The model under review builds one solid part; all positions refer to its coordinate system, in mm. A direction names the side the tool comes from. Coordinates: 2 decimals unless noted, no trailing zeros. Write each loop counter-clockwise with the first axis right and the second up, starting at its lowest first coordinate (ties: lowest second). Pieces come first, ordered by that corner, then holes. Notation, with made-up numbers: M -37,10.25 L 22,10.25 A15 ccw 22,18.25 Z; hole C 24,28 d9. An arc over 180 degrees is marked long. Answer as CSV lines item,"result". Start each with the question number.
Autodesk Inventor part; units mm, degrees
ref_plane "YZ Plane" through (0, 0, 0) normal (1, 0, 0) x (0, 1, 0)
ref_plane "XZ Plane" through (0, 0, 0) normal (0, 1, 0) x (-1, 0, 0)
ref_plane "XY Plane" through (0, 0, 0) normal (0, 0, 1) x (1, 0, 0)
sketch "Szkic1" plane through (0, 0, 0) normal (0, 1, 0) x (-1, 0, 0)
  line L0 (1.5, 2) -> (-1.5, 2)
  line L1 (-1.5, 2) -> (-1.5, -2)
  line L2 (-1.5, -2) -> (1.5, -2)
  line L3 (1.5, -2) -> (1.5, 2)
  line L4 (1.5, 2) -> (-1.5, -2) construction
  line L5 (-1.5, 2) -> (1.5, -2) construction
  point P0 (0, 0)
  dimension "d0" = 4
  dimension "d1" = 3
extrude "Wyciągnięcie proste1" add sketch "Szkic1" along normal blind 26.5
sketch "Szkic2" plane through (-1.5, 0, -2) normal (-1, 0, 0) x (0, 0, 1)
  line L0 (4, 26.5) -> (0, 26.5)
  line L1 (4, 0) -> (4, 26.5)
  line L2 (0, 26.5) -> (4, 26.5)
  line L3 (4, 26.5) -> (4, 22.5)
  line L4 (4, 22.5) -> (0, 22.5)
  line L5 (0, 22.5) -> (0, 26.5)
  point P0 (2, 0)
  dimension "d4" = 4
extrude "Wyciągnięcie proste2" add sketch "Szkic2" along normal blind 15.5
sketch "Szkic3" plane through (-1.5, 22.5, -2) normal (0, -1, 0) x (1, 0, 0)
  line L0 (3, 4) -> (-15.5, 4)
  line L1 (3, 0) -> (-15.5, 0)
  line L2 (-15.5, 4) -> (-12.5, 4)
  line L3 (-12.5, 4) -> (-12.5, 0)
  line L4 (-12.5, 0) -> (-15.5, 0)
  line L5 (-15.5, 0) -> (-15.5, 4)
  point P0 (1.5, 2)
  dimension "d7" = 3
extrude "Wyciągnięcie proste3" add sketch "Szkic3" along normal blind 22.5
sketch "Szkic4" plane through (1.5, 0, 2) normal (1, 0, 0) x (0, 0, -1)
  line L0 (4, 0) -> (0, 0)
  line L1 (4, 22.5) -> (4, 0)
  line L2 (0, 0) -> (4, 0)
  line L3 (4, 0) -> (4, 3)
  line L4 (4, 3) -> (0, 3)
  line L5 (0, 3) -> (0, 0)
  point P0 (2, 0)
  dimension "d10" = 3
extrude "Wyciągnięcie proste4" add sketch "Szkic4" along normal blind 4
sketch "Szkic5" plane through (-17, 0, -2) normal (-1, 0, 0) x (0, 0, 1)
  line L0 (0, 0) -> (4, 0)
  line L1 (4, 3) -> (0, 3)
  line L2 (0, 0) -> (4, 0)
  line L3 (4, 0) -> (4, 3)
  line L4 (4, 3) -> (0, 3)
  line L5 (0, 3) -> (0, 0)
  point P0 (2, 0)
extrude "Wyciągnięcie proste5" add sketch "Szkic5" along normal blind 4
sketch "Szkic6" plane through (1.5, 3, 2) normal (0, 1, 0) x (1, 0, 0)
  line L0 (0, 0) -> (4, 0)
  line L1 (0, 4) -> (4, 4)
  line L2 (4, 0) -> (0, 4)
  line L3 (4, 0) -> (4, 4)
  line L4 (0, 0) -> (4, 4)
  circle A0 centre (2, 2) radius 1.1
  line L5 (-22.5, 4) -> (-22.5, 0)
  line L6 (-18.5, 4) -> (-18.5, 0)
  line L7 (-22.5, 0) -> (-18.5, 4)
  line L8 (-18.5, 4) -> (-22.5, 4)
  line L9 (-18.5, 0) -> (-22.5, 4)
  circle A1 centre (-20.5, 2) radius 1.1
  point P0 (-1.5, 2)
  dimension "d15" = 2.2
  dimension "d16" = 2.2
hole "Otwór1" at (3.5, 3, 0) at (-19, 3, 0) direction (0, -1, 0) diameter 2.2 end through all
sketch "Szkic7" plane through (1.5, 26.5, -2) normal (0, 0, -1) x (-1, 0, 0)
  line L0 (3, -4) -> (15.5, -4)
  line L1 (3, -4) -> (3, 0)
  line L2 (0, 0) -> (18.5, 0)
  line L3 (15.5, -4) -> (15.5, -26.5)
  line L4 (3, 0) -> (15.5, -4)
  line L5 (15.5, -4) -> (15.5, 0)
  line L6 (15.5, 0) -> (3, -4)
  point P0 (1.5, -26.5)
  point P1 (9.25, -2)
hole "Otwór3" at (-7.75, 24.5, -2) direction (0, 0, 1) diameter 2.2 end through all
properties part number "mocowanie-serwomechanizmy"
1) Take a section at B-B on z = 0. Give the boundary of the cut face in (x, y).
2) Mouldability with a two-part tool opening along X and no side actions: class faces 5 (the flat face through (2, 0, 0)), 6 (the cylindrical face through (-17.926, 1.479, -0.238)), 7 (the flat face through (-17, 15, 0)), 8 (the flat face through (-1.5, 11, 0)) as +X half, -X half, draft (parallel to the pull), parting line (faces both ways), or undercut.
3) To check wall thickness, follow line 1 (X direction, y = 1.9, z = 0); line 2 (X direction, y = 7.25, z = -1.05); line 3 (Z direction, x = 3.5, y = 1). State the ranges of each line that lie inside material, in increasing order. Write a range as [from, to].
4) Take a section at D-D on z = 1.5. Give the boundary of the cut face in (x, y).
5) Take a section at C-C on x = -7.75. Give the boundary of the cut face in (y, z).
6) Take a section at A-A on y = 12.5. Give the boundary of the cut face in (x, z).
7) Tool access review of faces 1 (the flat face through (-20, 3, 1)), 2 (the flat face through (-8, 22.5, 0)), 3 (the flat face through (1.5, 15, 0)), 4 (the cylindrical face through (2.41, 1.48, -0.14)): name each direction out of +Z, -Z, +X, -X, +Y, -Y from which nothing blocks a thin tool from reaching the whole face with its end or side.
8) Clearance check with flat-ended pins moving along their axes: pin 1 Ø6 at (x, y) = (-2, 20) entering from -Z; pin 2 Ø1.2 at (x, z) = (-20, 0) entering from +Y; pin 3 Ø1.5 at (y, z) = (5, 0.5) entering from +X. State where each tip first meets the part, or that it passes through.
Results:
1,outline,"M -21,0 L -20.1,0 L -20.1,3 L -21,3 Z; M -17.9,0 L -14,0 L -14,22.5 L -1.5,22.5 L -1.5,0 L 2.4,0 L 2.4,3 L 1.5,3 L 1.5,26.5 L -17,26.5 L -17,3 L -17.9,3 Z; M 4.6,0 L 5.5,0 L 5.5,3 L 4.6,3 Z; hole C -7.75,24.5 d2.2"
2,face 5,"draft"
2,face 6,"undercut"
2,face 7,"-X half"
2,face 8,"undercut"
3,line 1,"x = [-21, -20.1], [-17.9, -14], [-1.5, 2.4], [4.6, 5.5]"
3,line 2,"x = [-17, -14], [-1.5, 1.5]"
3,line 3,"z = [-2, -1.1], [1.1, 2]"
4,outline,"M -21,0 L -14,0 L -14,22.5 L -1.5,22.5 L -1.5,0 L 5.5,0 L 5.5,3 L 1.5,3 L 1.5,26.5 L -17,26.5 L -17,3 L -21,3 Z; hole C -7.75,24.5 d2.2"
5,outline,"M 22.5,-2 L 23.4,-2 L 23.4,2 L 22.5,2 Z; M 25.6,-2 L 26.5,-2 L 26.5,2 L 25.6,2 Z"
6,outline,"M -17,-2 L -14,-2 L -14,2 L -17,2 Z; M -1.5,-2 L 1.5,-2 L 1.5,2 L -1.5,2 Z"
7,face 1,"+Z, -Z, -X, +Y"
7,face 2,"+Z, -Z, -Y"
7,face 3,"+Z, -Z, +X, +Y"
7,face 4,"+Y, -Y"
8,pin 1,"stops at z = -2"
8,pin 2,"stops at y = 3"
8,pin 3,"stops at x = 1.5"
